The listing builds one solid part. Answer for the finished solid, in the listing's coordinates (mm). Round coordinates to 2 decimals unless told otherwise and drop trailing zeros. Write each loop counter-clockwise with the first axis right and the second up, starting at its lowest first coordinate (ties: lowest second). Pieces come first, ordered by that corner, then holes. Notation, with made-up numbers: (-30, 6.25) - (-13, 6.25) arc R18 cw to (-13, 25.25) - close; hole circle Ø6 at (8.5, -21.5). An arc over 180 degrees is marked (long way). Answer in a Markdown table with one row per item.
from build123d import *

# Parameters (mm, degrees)
SKIZZE1_W                       = 20
SKIZZE1_H                       = 350
AUFSATZ_LINEAR_AUSTRAGEN1_DEPTH = 5
SKIZZE2_R                       = 3
SCHNITT_LINEAR_AUSTRAGEN1_DEPTH = 10
LINEARES_MUSTER1_COUNT          = 6
LINEARES_MUSTER1_PITCH          = 60


with BuildPart() as part:
    # Skizze1 → Aufsatz-Linear austragen1 (new body)
    with BuildSketch(Plane.XY):
        with Locations((0, 175)):
            Rectangle(SKIZZE1_W, SKIZZE1_H)
    extrude(amount=AUFSATZ_LINEAR_AUSTRAGEN1_DEPTH)

    # Skizze2 → Schnitt-Linear austragen1 (cut)
    with BuildSketch(Plane.XY.offset(5)):
        with Locations((0, 20)):
            Circle(SKIZZE2_R)
    schnitt_linear_austragen1 = extrude(amount=-SCHNITT_LINEAR_AUSTRAGEN1_DEPTH, mode=Mode.SUBTRACT)

    # Lineares Muster1: Schnitt-Linear austragen1 ×6
    with Locations(*[(0, i * LINEARES_MUSTER1_PITCH, 0) for i in range(1, LINEARES_MUSTER1_COUNT)]):
        add(schnitt_linear_austragen1, mode=Mode.SUBTRACT)


solid = part.part
(1) Find the intervals of material crossed by line 1 (X direction, y = 200, z = 1.85), in increasing order.
Checked values:
| item | result |
|---|---|
| line 1 | x = -10 to -3, 3 to 10 |
(2) Section C-C (y = 20) is taken. Give the vertices of the cut face in (x, z).
Checked values:
| item | result |
|---|---|
| outline | (-10, 0) - (-3, 0) - (-3, 5) - (-10, 5) - close; (3, 0) - (10, 0) - (10, 5) - (3, 5) - close |
(3) Section B-B (z = 1.8) is taken. Give the vertices of the cut face in (x, y).
Checked values:
| item | result |
|---|---|
| outline | (-10, 0) - (10, 0) - (10, 350) - (-10, 350) - close; hole circle Ø6 at (0, 20); hole circle Ø6 at (0, 80); hole circle Ø6 at (0, 140); hole circle Ø6 at (0, 200); hole circle Ø6 at (0, 260); hole circle Ø6 at (0, 320) |
(4) Section A-A (x = 0) is taken. Give the vertices of the cut face in (y, z).
Checked values:
| item | result |
|---|---|
| outline | (0, 0) - (17, 0) - (17, 5) - (0, 5) - close; (23, 0) - (77, 0) - (77, 5) - (23, 5) - close; (83, 0) - (137, 0) - (137, 5) - (83, 5) - close; (143, 0) - (197, 0) - (197, 5) - (143, 5) - close; (203, 0) - (257, 0) - (257, 5) - (203, 5) - close; (263, 0) - (317, 0) - (317, 5) - (263, 5) - close; (323, 0) - (350, 0) - (350, 5) - (323, 5) - close |
(5) For a pull along X with two mould halves and no side action, classify faces 1 (the flat face through (0, 177, 5)), 2 (the cylindrical face through (1.61, 142.53, 2.54)), 3 (the cylindrical face through (0, 203, 3)) as pulls with the +X half, pulls with the -X half, needs draft (parallel to the pull), parting line crosses it, or undercut.
Checked values:
| item | result |
|---|---|
| face 1 | needs draft |
| face 2 | undercut |
| face 3 | undercut |
